The listing builds one solid part. Answer for the finished solid, in the listing's coordinates (mm). Coordinates: 2 decimals unless noted, no trailing zeros. Write each loop counter-clockwise with the first axis right and the second up, starting at its lowest first coordinate (ties: lowest second). Pieces come first, ordered by that corner, then holes. Notation, with made-up numbers: M 89.5,-24.5 L 137.5,-24.5 A19 ccw 137.5,-5.5 Z; hole C 85.5,61 d8. An arc over 180 degrees is marked long. Answer as a JSON object with one key per item and string values. Group by question number.
from build123d import *

# Parameters (mm, degrees)
SKETCH1_W           = 330.2
SKETCH1_H           = 57.15
BOSS_EXTRUDE1_DEPTH = 6.35
SKETCH3_W           = 24.892
SKETCH3_H           = 18.542
BOSS_EXTRUDE2_DEPTH = 6.35
SKETCH4_W           = 13.208
SKETCH4_H           = 13.208
CUT_EXTRUDE2_DEPTH  = 172.809034073


with BuildPart() as part:
    # Sketch1 → Boss-Extrude1 (new body)
    with BuildSketch(Plane(origin=(0, 0, 0), x_dir=(1, 0, 0), z_dir=(0, 1, 0))):
        Rectangle(SKETCH1_W, SKETCH1_H)
    extrude(amount=BOSS_EXTRUDE1_DEPTH)

    # Sketch3 → Boss-Extrude2 (add)
    with BuildSketch(Plane(origin=(0, 0, 0), x_dir=(1, 0, 0), z_dir=(0, 1, 0))):
        with Locations((-114.3, -37.846)):
            Rectangle(SKETCH3_W, SKETCH3_H)
        with Locations((-76.2, -37.846)):
            Rectangle(SKETCH3_W, SKETCH3_H)
        with Locations((-38.1, -37.846)):
            Rectangle(SKETCH3_W, SKETCH3_H)
        with Locations((0, -37.846)):
            Rectangle(SKETCH3_W, SKETCH3_H)
        with Locations((38.1, -37.846)):
            Rectangle(SKETCH3_W, SKETCH3_H)
        with Locations((76.2, -37.846)):
            Rectangle(SKETCH3_W, SKETCH3_H)
        with Locations((114.3, -37.846)):
            Rectangle(SKETCH3_W, SKETCH3_H)
        with Locations((152.4, -37.846)):
            Rectangle(SKETCH3_W, SKETCH3_H)
        with Locations((-152.4, -37.846)):
            Rectangle(SKETCH3_W, SKETCH3_H)
    extrude(amount=BOSS_EXTRUDE2_DEPTH)

    # Sketch4 → Cut-Extrude2 (cut, through all)
    with BuildSketch(Plane(origin=(0, 0, 0), x_dir=(1, 0, 0), z_dir=(0, 1, 0))):
        with Locations((165.1, 22.225)):
            Rectangle(SKETCH4_W, SKETCH4_H)
        with Locations((-165.1, -28.575)):
            Rectangle(SKETCH4_W, SKETCH4_H)
        with Locations((165.1, -3.175)):
            Rectangle(SKETCH4_W, SKETCH4_H)
        with Locations((165.1, -28.575)):
            Rectangle(SKETCH4_W, SKETCH4_H)
        with Locations((-165.1, -3.175)):
            Rectangle(SKETCH4_W, SKETCH4_H)
        with Locations((-165.1, 22.225)):
            Rectangle(SKETCH4_W, SKETCH4_H)
    extrude(amount=CUT_EXTRUDE2_DEPTH, mode=Mode.SUBTRACT)


solid = part.part
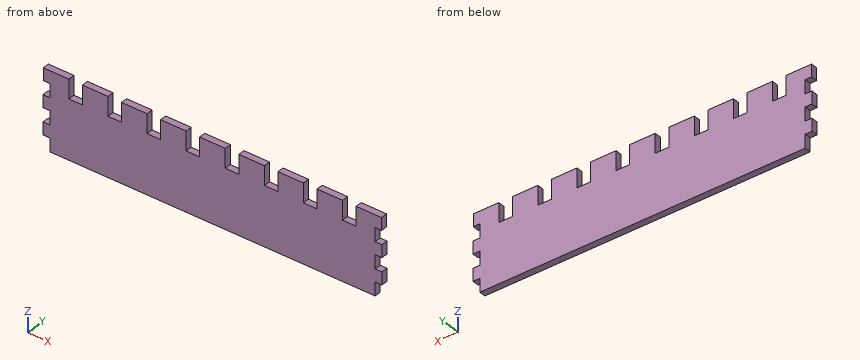
Item 1: A cutting plane is placed at A-A, the plane x = -131. Write down the section's boundary in (y, z) (3 decimals), and give its area (3 significant figures).
Item 2: Flat-ended cylindrical pins translate along their axes: pin 1 Ø3 at (y, z) = (3.5, 40.5) entering from +X; pin 2 Ø1.9 at (x, y) = (161.5, 2.5) entering from -Z; pin 3 Ø1.9 at (x, y) = (54.5, 1.5) entering from +Z (3 decimals). Find the tip coordinate at first contact, or state that the pin passes through.
Item 3: Consider L1, parallel to X at y = 1.25, z = 23.5. Determine where the line is inside the solid, lowest interval first. Write a range as from..to.
Item 4: A cutting plane is placed at B-B, the plane z = -0.5. Write down the section's boundary in (x, y).
Answer:
{
 "1": {"outline": "M 0,-28.575 L 6.35,-28.575 L 6.35,28.575 L 0,28.575 Z", "area": "363 mm2"},
 "2": {"pin 1": "x = 164.85", "pin 2": "z = -15.62", "pin 3": "z = 28.575"},
 "3": {"L1": "-158.5..158.5"},
 "4": {"outline": "M -158.5,0 L 158.5,0 L 158.5,6.35 L -158.5,6.35 Z"}
}
